The model under review builds one solid part; all positions refer to its coordinate system, in mm. Face numbers are marked on the shaded views. A direction names the side the tool comes from. Give positions to 0.01 mm unless a question says otherwise; leave off trailing zeros. Loops run counter-clockwise (first coordinate to the right, second up) from the corner with the lowest first, then second, coordinate; pieces in that order, holes last. Notation, with made-up numbers: (28, -24) - (60, -24) arc R25 cw to (60, -9) - close; hole circle Ø2 at (48, 8.5). An arc over 180 degrees is marked (long way). Answer as a JSON object with one key per item and string values.
from build123d import *

# Parameters (mm, degrees)
SKETCH2_W           = 54
SKETCH2_H           = 162
SKETCH2_R           = 10.5
BOSS_EXTRUDE1_DEPTH = 12
SKETCH3_W           = 18
SKETCH3_H           = 12
BOSS_EXTRUDE2_DEPTH = 12
CUT_EXTRUDE1_REACH  = 99.581
SKETCH4_R           = 2.25
LPATTERN1_COUNT     = 3
LPATTERN1_PITCH     = 45
CUT_EXTRUDE2_DEPTH  = 6
LPATTERN2_COUNT     = 2
LPATTERN2_PITCH     = 45
LPATTERN2_COL_COUNT = 2
LPATTERN2_COL_PITCH = 45
CUT_EXTRUDE3_REACH  = 99.581
SKETCH6_R           = 5
SKETCH8_R           = 5
CUT_EXTRUDE4_DEPTH  = 6
CUT_EXTRUDE5_REACH  = 99.026
SKETCH9_R           = 3
SKETCH10_R          = 3
CUT_EXTRUDE6_DEPTH  = 19
CUT_EXTRUDE7_REACH  = 99.581
SKETCH11_R          = 3
CUT_EXTRUDE8_DEPTH  = 6


with BuildPart() as part:
    # Sketch2 → Boss-Extrude1 (new body)
    with BuildSketch(Plane(origin=(0, 0, 0), x_dir=(0, 0, -1), z_dir=(1, 0, 0))):
        Rectangle(SKETCH2_W, SKETCH2_H)
        Circle(SKETCH2_R, mode=Mode.SUBTRACT)
        with Locations((0, 45)):
            Circle(SKETCH2_R, mode=Mode.SUBTRACT)
        with Locations((0, -45)):
            Circle(SKETCH2_R, mode=Mode.SUBTRACT)
    extrude(amount=BOSS_EXTRUDE1_DEPTH)

    # Sketch3 → Boss-Extrude2 (add)
    with BuildSketch(Plane(origin=(12, 0, 0), x_dir=(0, 0, -1), z_dir=(1, 0, 0))):
        with Locations((0, -87)):
            Rectangle(SKETCH3_W, SKETCH3_H)
    boss_extrude2 = extrude(amount=-BOSS_EXTRUDE2_DEPTH)

    # Mirror1: Boss-Extrude2 across plane
    add(boss_extrude2.mirror(Plane.ZX))

    # Sketch4 → Cut-Extrude1 (cut, up to next)
    with BuildSketch(Plane(origin=(12, 0, 0), x_dir=(0, 0, -1), z_dir=(1, 0, 0)), mode=Mode.PRIVATE) as cut_extrude1_sk1:
        with Locations((-16, -45)):
            Circle(SKETCH4_R)
    cut_extrude1_tool1 = extrude(cut_extrude1_sk1.sketch, amount=-CUT_EXTRUDE1_REACH, mode=Mode.PRIVATE) & part.part
    # Sketch4 → Cut-Extrude1 (cut, up to next)
    with BuildSketch(Plane(origin=(12, 0, 0), x_dir=(0, 0, -1), z_dir=(1, 0, 0)), mode=Mode.PRIVATE) as cut_extrude1_sk2:
        with Locations((16, -45)):
            Circle(SKETCH4_R)
    cut_extrude1_tool2 = extrude(cut_extrude1_sk2.sketch, amount=-CUT_EXTRUDE1_REACH, mode=Mode.PRIVATE) & part.part
    cut_extrude1_1 = cut_extrude1_tool1.solids().sort_by_distance((12, -45, 16))[0]
    add(cut_extrude1_1, mode=Mode.SUBTRACT)
    cut_extrude1_2 = cut_extrude1_tool2.solids().sort_by_distance((12, -45, -16))[0]
    add(cut_extrude1_2, mode=Mode.SUBTRACT)
    cut_extrude1 = cut_extrude1_1 + cut_extrude1_2  # Cut-Extrude1 as one shape, for the pattern or mirror that repeats it

    # LPattern1: Cut-Extrude1 ×3
    with Locations(*[(0, i * LPATTERN1_PITCH, 0) for i in range(1, LPATTERN1_COUNT)]):
        add(cut_extrude1, mode=Mode.SUBTRACT)

    # Sketch5 → Cut-Extrude2 (cut)
    with BuildSketch(Plane.ZY):
        with BuildLine():
            Line((-16.992645468, 15.5), (16.992645468, 15.5))
            ThreePointArc((16.992645468, 15.5), (23, 0), (16.992645468, -15.5))
            Line((16.992645468, -15.5), (-16.992645468, -15.5))
            ThreePointArc((-16.992645468, -15.5), (-23, 0), (-16.992645468, 15.5))
        make_face()
    cut_extrude2 = extrude(amount=-CUT_EXTRUDE2_DEPTH, mode=Mode.SUBTRACT)

    # LPattern2: Cut-Extrude2 ×2
    with Locations(*[(0, -i * LPATTERN2_PITCH, 0) for i in range(1, LPATTERN2_COUNT)]):
        add(cut_extrude2, mode=Mode.SUBTRACT)

    # LPattern2 col: Cut-Extrude2 ×2
    with Locations(*[(0, i * LPATTERN2_COL_PITCH, 0) for i in range(1, LPATTERN2_COL_COUNT)]):
        add(cut_extrude2, mode=Mode.SUBTRACT)

    # Sketch6 → Cut-Extrude3 (cut, up to next)
    with BuildSketch(Plane.ZY, mode=Mode.PRIVATE) as cut_extrude3_sk1:
        with Locations((-18, -69)):
            Circle(SKETCH6_R)
    cut_extrude3_tool1 = extrude(cut_extrude3_sk1.sketch, amount=-CUT_EXTRUDE3_REACH, mode=Mode.PRIVATE) & part.part
    # Sketch6 → Cut-Extrude3 (cut, up to next)
    with BuildSketch(Plane.ZY, mode=Mode.PRIVATE) as cut_extrude3_sk2:
        with Locations((18, -69)):
            Circle(SKETCH6_R)
    cut_extrude3_tool2 = extrude(cut_extrude3_sk2.sketch, amount=-CUT_EXTRUDE3_REACH, mode=Mode.PRIVATE) & part.part
    cut_extrude3_1 = cut_extrude3_tool1.solids().sort_by_distance((0, -69, -18))[0]
    add(cut_extrude3_1, mode=Mode.SUBTRACT)
    cut_extrude3_2 = cut_extrude3_tool2.solids().sort_by_distance((0, -69, 18))[0]
    add(cut_extrude3_2, mode=Mode.SUBTRACT)
    cut_extrude3 = cut_extrude3_1 + cut_extrude3_2  # Cut-Extrude3 as one shape, for the pattern or mirror that repeats it

    # Sketch8 → Cut-Extrude4 (cut)
    with BuildSketch(Plane.ZY):
        with Locations((0, -87)):
            Circle(SKETCH8_R)
    cut_extrude4 = extrude(amount=-CUT_EXTRUDE4_DEPTH, mode=Mode.SUBTRACT)

    # Sketch9 → Cut-Extrude5 (cut, up to next)
    with BuildSketch(Plane.ZY.offset(-6), mode=Mode.PRIVATE) as cut_extrude5_sk1:
        with Locations((0, -87)):
            Circle(SKETCH9_R)
    cut_extrude5_tool1 = extrude(cut_extrude5_sk1.sketch, amount=-CUT_EXTRUDE5_REACH, mode=Mode.PRIVATE) & part.part
    cut_extrude5 = cut_extrude5_tool1.solids().sort_by_distance((6, -87, 0))[0]
    add(cut_extrude5, mode=Mode.SUBTRACT)

    # Sketch10 → Cut-Extrude6 (cut)
    with BuildSketch(Plane.XZ.offset(81)):
        with Locations(Location((6, -18, 0), (0, 0, 270))):
            Circle(SKETCH10_R)
        with Locations(Location((6, 18, 0), (0, 0, 270))):
            Circle(SKETCH10_R)
    cut_extrude6 = extrude(amount=-CUT_EXTRUDE6_DEPTH, mode=Mode.SUBTRACT)

    # Sketch11 → Cut-Extrude7 (cut, up to next)
    with BuildSketch(Plane.ZY, mode=Mode.PRIVATE) as cut_extrude7_sk1:
        with Locations((-21, -22.5)):
            Circle(SKETCH11_R)
    cut_extrude7_tool1 = extrude(cut_extrude7_sk1.sketch, amount=-CUT_EXTRUDE7_REACH, mode=Mode.PRIVATE) & part.part
    cut_extrude7 = cut_extrude7_tool1.solids().sort_by_distance((0, -22.5, -21))[0]
    add(cut_extrude7, mode=Mode.SUBTRACT)

    # Sketch12 → Cut-Extrude8 (cut)
    with BuildSketch(Plane.ZY):
        with BuildLine():
            Line((-21, -27.5), (-27, -27.5))
            Line((-27, -27.5), (-27, -17.5))
            Line((-27, -17.5), (-21, -17.5))
            ThreePointArc((-21, -17.5), (-16, -22.5), (-21, -27.5))
        make_face()
    cut_extrude8 = extrude(amount=-CUT_EXTRUDE8_DEPTH, mode=Mode.SUBTRACT)

    # Mirror2: Cut-Extrude3, Cut-Extrude4, Cut-Extrude5, Cut-Extrude6, Cut-Extrude7, Cut-Extrude8 across plane
    add(cut_extrude3.mirror(Plane.ZX), mode=Mode.SUBTRACT)
    add(cut_extrude4.mirror(Plane.ZX), mode=Mode.SUBTRACT)
    add(cut_extrude5.mirror(Plane.ZX), mode=Mode.SUBTRACT)
    add(cut_extrude6.mirror(Plane.ZX), mode=Mode.SUBTRACT)
    add(cut_extrude7.mirror(Plane.ZX), mode=Mode.SUBTRACT)
    add(cut_extrude8.mirror(Plane.ZX), mode=Mode.SUBTRACT)


solid = part.part
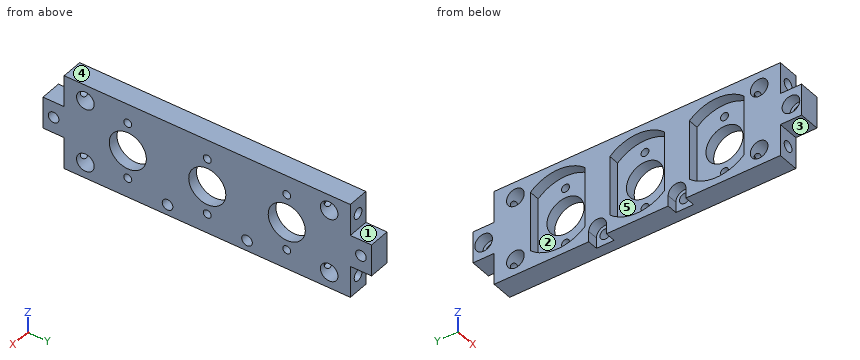
Q1. For the marked faces 1, 2 and 3, list the 3-axis set-ups (+Z, -Z, +X, -X, +Y, -Y) from which the entire face can be reached by the end or side of a thin tool; tool diameter is ignored.
Results:
{"face 1": "+Z, +X, -X, +Y", "face 2": "-X", "face 3": "-Z, +X, -X, -Y"}
Q2. Clearance check with flat-ended pins moving along their axes: pin 1 Ø5 at (x, z) = (4, -25) entering from -Y; pin 2 Ø8 at (y, z) = (-89, -1) entering from -X; pin 3 Ø1.8 at (x, z) = (7.5, -17) entering from -Y; pin 4 Ø6 at (x, z) = (8, -17) entering from +Y. State where each tip first meets the part, or that it passes through.
Results:
{"pin 1": "stops at y = -81", "pin 2": "stops at x = 0", "pin 3": "stops at y = -62", "pin 4": "stops at y = 81"}
Q3. Consider section A-A, the plane y = 45. State the section outline as (x, z) points.
Results:
{"outline": "(0, -27) - (12, -27) - (12, -18.25) - (6, -18.25) - (6, -23) - (0, -23) - close; (0, 23) - (6, 23) - (6, 18.25) - (12, 18.25) - (12, 27) - (0, 27) - close; (6, -13.75) - (12, -13.75) - (12, -10.5) - (6, -10.5) - close; (6, 10.5) - (12, 10.5) - (12, 13.75) - (6, 13.75) - close"}
Q4. The part is to be moulded in two halves that separate along Y. For the marked faces 4 and 5, say which applies: +Y half, -Y half, draft (parallel to the pull), parting line (faces both ways), or undercut.
Results:
{"face 4": "draft", "face 5": "undercut"}
Q5. To check wall thickness, follow probe 1 along Y at (x, z) = (1, 15); probe 2 along Y at (x, z) = (9.45, 0); probe 3 along Z at (x, y) = (6, 63.9). State the ranges of each line that lie inside material, in increasing order. Write a range as [from, to].
Results:
{"probe 1": "y = [-81, -73], [-65, -60.5], [-29.5, -15.5], [15.5, 29.5], [60.5, 65], [73, 81]", "probe 2": "y = [-93, -90], [-84, -55.5], [-34.5, -10.5], [10.5, 34.5], [55.5, 84], [90, 93]", "probe 3": "z = [-27, -21], [-15, 15], [21, 27]"}
Q6. Consider section B-B, the plane y = -22.5. State the section outline as (x, z) points, plus the area to 3 significant figures.
Results:
{"outline": "(0, -16) - (6, -16) - (6, -18) - (12, -18) - (12, 27) - (0, 27) - close; (6, -27) - (12, -27) - (12, -24) - (6, -24) - close", "area": "546 mm^2"}
